Autodesk Inventor part; units mm, degrees
ref_plane "Work Plane1" through (14.605, 0, 0) normal (1, 0, 0) x (0, 0, -1)
ref_plane "Work Plane2" through (-3.175, 0, 0) normal (-1, 0, 0) x (0, 0, 1)
ref_plane "YZ Plane" through (0, 0, 0) normal (1, 0, 0) x (0, 1, 0)
sketch "Sketch1" plane through (0, 0, 0) normal (1, 0, 0) x (0, 1, 0)
  circle A0 centre (0, 0) radius 6.477
  dimension "d0" = 12.954
extrude "Extrusion1" add sketch "Sketch1" along normal blind 11.43
sketch "Sketch2" plane through (11.43, 0, 0) normal (1, 0, 0) x (0, 0, -1)
  circle A0 centre (0, 0) radius 6.477
ref_plane "Work Plane1" through (14.605, 0, 0) normal (1, 0, 0) x (0, 0, -1)
sketch "Sketch3" plane through (14.605, 0, 0) normal (1, 0, 0) x (0, 0, -1)
  circle A0 centre (0, 0) radius 3.302
  dimension "d4" = 6.604
loft "Loft1" add profiles "Sketch3" section 2 edges at (11.43, -6.477, 0)
ref_plane "Work Plane2" through (-3.175, 0, 0) normal (-1, 0, 0) x (0, 0, 1)
sketch "Sketch4" plane through (-3.175, 0, 0) normal (-1, 0, 0) x (0, 0, 1)
  circle A0 centre (0, 0) radius 3.302
  dimension "d10" = 6.604
loft "Loft2" add profiles "Sketch4" section 2 edges at (0, -6.477, 0)
properties part number "shaft 6x24"
The listing builds one solid part. Answer for the finished solid, in the listing's coordinates (mm). Give positions to 0.01 mm unless a question says otherwise; leave off trailing zeros. Write each loop counter-clockwise with the first axis right and the second up, starting at its lowest first coordinate (ties: lowest second). Pieces come first, ordered by that corner, then holes. Notation, with made-up numbers: (-14, -13.75) - (30, -13.75) arc R29 ccw to (30, 17.25) - close; hole circle Ø5 at (-36.75, -34.75). An arc over 180 degrees is marked (long way). Use one line per item in the form item = value. Start each with the question number.
1) Consider line 1 along Z through (x, y) = (6, -1.5); line 2 along Y through (x, z) = (5.75, -4.5); line 3 along Z through (x, y) = (-0.5, 4). Determine where each line is inside the solid, lowest interval first. Write a range as from..to.
2) Find section B-B on x = 0.75. Determine the outline of the cut face in (y, z).
3) Find section A-A on z = 0. Determine the outline of the cut face in (x, y) (3 decimals), plus the area to 3 significant figures.
4) Find section C-C on x = 13.25. Determine the outline of the cut face in (y, z).
5) Flat-ended cylindrical pins translate along their axes: pin 1 Ø5 at (x, z) = (1.5, 1) entering from +Y; pin 2 Ø3 at (x, y) = (7, -2.5) entering from -Z. Find the tip coordinate at first contact, or state that the pin passes through.
Geometry results:
q1.line_1 = -6.3..6.3
q1.line_2 = -4.66..4.66
q1.line_3 = -4.44..4.44
q2.outline = circle Ø12.95 at (0, 0)
q3.outline = (-3.175, -3.302) - (0, -6.477) - (11.43, -6.477) - (14.605, -3.302) - (14.605, 3.302) - (11.43, 6.477) - (0, 6.477) - (-3.175, 3.302) - close
q3.area = 210 mm2
q4.outline = circle Ø9.31 at (0, 0)
q5.pin_1 = 6.48
q5.pin_2 = -6.4
